Autodesk Fusion 360 part; units mm, degrees
sketch "Sketch1" plane through (0, 0, 0) normal (0, 0, 1) x (1, 0, 0)
  circle A0 centre (0, 0) radius 5.5
  dimension "d3" = 11
extrude "Extrude1" add sketch "Sketch1" along normal blind 1.8
sketch "Sketch2" plane through (0, 0, 1.8) normal (0, 0, 1) x (-1, 0, 0)
  circle A0 centre (0, 0) radius 5.5
  circle A1 centre (0, 0) radius 2.3
  dimension "d6" = 4.6
extrude "Extrude2" add sketch "Sketch2" along normal blind 2.2 contours A1
chamfer "Chamfer1" distance 0.6 angle 45 1 edges at (-5.1278, -1.9889, 0)
Could you check a few things on this model? Use its own coordinates, in mm. Give positions to 0.01 mm unless a question says otherwise; leave off trailing zeros. Order: outer loops, then holes, each group sorted by start corner. A loop starts at its lowest first (then second) coordinate and runs counter-clockwise, first axis right, second up. Notation, with made-up numbers: (-36.5, -6) - (-29.5, -6) arc R23 ccw to (-29.5, 18) - close; hole circle Ø8 at (0.5, 26.5). An arc over 180 degrees is marked (long way). One line per question, with ' | ' between items. Start each with the question number.
Item 1: I'm going to push a flat-ended pin straight in: pin 1 Ø2 at (y, z) = (1, 3) entering from -X. Where does the tip first touch, or does it pass through?
Item 2: I need wall thicknesses on probe 1 along Z at (x, y) = (0.25, -3.75); probe 2 along Y at (x, z) = (2.5, 1.05); probe 3 along Y at (x, z) = (4, 1.6). Which ranges of each line are inside material? Lowest first, please. Write a range as [from, to].
Item 3: I want a section at A-A on y = 0. Write out the boundary of the cut face in (x, z).
Item 4: I want a section at D-D on z = 2.45. Write out the boundary of the cut face in (x, y), then the cut area to 3 significant figures.
Item 5: I want a section at C-C on z = 0.45. Write out the boundary of the cut face in (x, y), then the cut area to 3 significant figures.
Item 6: Thinking about a two-plate mould opening in Z: for faces 1 (the cylindrical face through (1.825, -1.4, 2.885)), 2 (the flat face through (0, 0, 0)), 3 (the flat face through (1.1, -2.4, 1.8)), which applies, pulls with the +Z half, pulls with the -Z half, needs draft (parallel to the pull), parting line crosses it, or undercut?
Verdict:
1) pin 1: x = -2.3
2) probe 1: [0, 1.8] | probe 2: [-4.9, 4.9] | probe 3: [-3.77, 3.77]
3) outline: (-5.5, 0.6) - (-4.9, 0) - (4.9, 0) - (5.5, 0.6) - (5.5, 1.8) - (2.3, 1.8) - (2.3, 4) - (-2.3, 4) - (-2.3, 1.8) - (-5.5, 1.8) - close
4) outline: circle Ø4.6 at (0, 0) | area: 16.6 mm^2
5) outline: circle Ø10.7 at (0, 0) | area: 89.9 mm^2
6) face 1: needs draft | face 2: pulls with the -Z half | face 3: pulls with the +Z half
